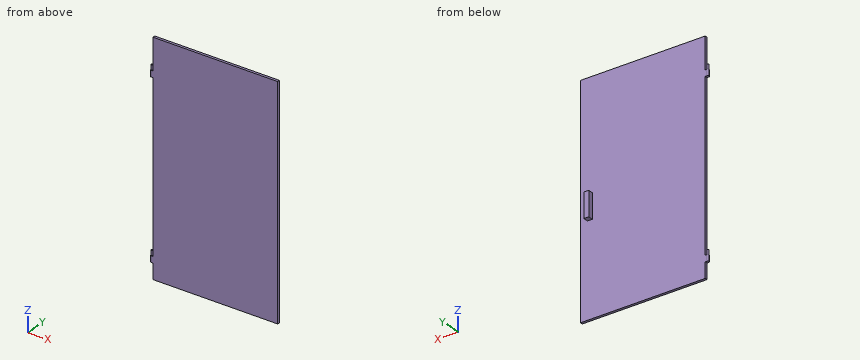
from build123d import *

# Parameters (mm, degrees)
SKETCH1_W           = 505
SKETCH1_H           = 915
BOSS_EXTRUDE1_DEPTH = 10
SKETCH2_W           = 25
SKETCH2_H           = 10
BOSS_EXTRUDE2_DEPTH = 12.5
SKETCH3_R           = 3.5
BOSS_EXTRUDE3_DEPTH = 20
LPATTERN1_COUNT     = 2
LPATTERN1_PITCH     = 700
FILLET1_R           = 5
SKETCH4_W           = 20
SKETCH4_H           = 100
BOSS_EXTRUDE4_DEPTH = 20


with BuildPart() as part:
    # Sketch1 → Boss-Extrude1 (new body)
    with BuildSketch(Plane(origin=(0, 0, 0), x_dir=(1, 0, 0), z_dir=(0, 1, 0))):
        with Locations((-7.5, -32.5)):
            Rectangle(SKETCH1_W, SKETCH1_H)
    extrude(amount=BOSS_EXTRUDE1_DEPTH)

    # Sketch2 → Boss-Extrude2 (add)
    with BuildSketch(Plane.ZY.offset(260)):
        with Locations((-350, 5)):
            Rectangle(SKETCH2_W, SKETCH2_H)
        with Locations((350, 5)):
            Rectangle(SKETCH2_W, SKETCH2_H)
    extrude(amount=BOSS_EXTRUDE2_DEPTH)

    # Sketch3 → Boss-Extrude3 (add)
    with BuildSketch(Plane.XY.offset(-337.5)):
        with Locations(Location((-267.5, 5, 0), (0, 0, 180))):
            Circle(SKETCH3_R)
    boss_extrude3 = extrude(amount=BOSS_EXTRUDE3_DEPTH)

    # LPattern1: Boss-Extrude3 ×2
    with Locations(*[(0, 0, i * LPATTERN1_PITCH) for i in range(1, LPATTERN1_COUNT)]):
        add(boss_extrude3)

    # Fillet1
    fillet1_edges = [part.edges().sort_by_distance(p)[0] for p in [
        (-272.5, 0, 350),
        (-272.5, 10, 350),
        (-272.5, 0, -350),
        (-272.5, 10, -350),
    ]]
    fillet(fillet1_edges, radius=FILLET1_R - 0.0001)  # a hair under: the kernel refuses the full size

    # Sketch4 → Boss-Extrude4 (add)
    with BuildSketch(Plane(origin=(0, 10, 0), x_dir=(1, 0, 0), z_dir=(0, 1, 0))):
        with Locations((206.961175434, 0)):
            Rectangle(SKETCH4_W, SKETCH4_H)
    extrude(amount=BOSS_EXTRUDE4_DEPTH)


solid = part.part
Here's how the part is built. I have some questions about the finished solid (model axes, mm). Coordinates: 2 decimals unless noted, no trailing zeros. Loops run counter-clockwise (first coordinate to the right, second up) from the corner with the lowest first, then second, coordinate; pieces in that order, holes last. Notation, with made-up numbers: (3.5, 9.5) -> (14.5, 9.5) arc R20 cw to (14.5, 29.5) -> close; hole circle Ø3 at (29.25, 60). An arc over 180 degrees is marked (long way). Use one line per item in the form item = value. Start each with the question number.
(1) Will these pins go through, and if not, where does the flat tip stop? pin 1 (5 mm diameter, centred on y = 7.5, z = 406, fed in from -X); pin 2 (3 mm diameter, centred on x = -268, y = 6, fed in from -Z); pin 3 (5 mm diameter, centred on y = 14, z = -156, fed in from -X); pin 4 (3 mm diameter, centred on x = -268, y = 6, fed in from +Z).
(2) If we section it at B-B (y = 18.25): Please give me the cut outline in (x, z).
(3) If we section it at C-C (x = 179.5): Please give me the cut outline in (y, z).
(4) Please list where these lines run through material, in increasing order: line 1 along Y through (x, z) = (86, -326); line 2 along X through (y, z) = (18, -22); line 3 along X through (y, z) = (5.5, -291).
(5) If we section it at A-A (z = -38): Please give me the cut outline in (x, y).
Verdict:
q1.pin_1 = -260
q1.pin_2 = -362.5
q1.pin_3 = through
q1.pin_4 = 382.5
q2.outline = (196.96, -50) -> (216.96, -50) -> (216.96, 50) -> (196.96, 50) -> close
q3.outline = (0, -425) -> (10, -425) -> (10, 490) -> (0, 490) -> close
q4.line_1 = 0 to 10
q4.line_2 = 196.96 to 216.96
q4.line_3 = -260 to 245
q5.outline = (-260, 0) -> (245, 0) -> (245, 10) -> (216.96, 10) -> (216.96, 30) -> (196.96, 30) -> (196.96, 10) -> (-260, 10) -> close
